from build123d import *

# Parameters (mm, degrees)
SKETCH1_W             = 10
SKETCH1_H             = 10
BOSS_EXTRUDE1_DEPTH   = 2.5
BOSS_EXTRUDE1_2_DEPTH = 2.5
BOSS_EXTRUDE2_DEPTH   = 3
F_2_CLEARANCE_HOLE1_D = 2.9464
FILLET1_R             = 2.5
F_2_CLEARANCE_HOLE2_D = 2.9464
CUT_EXTRUDE1_DEPTH    = 66.097235732
FILLET2_R             = 1
FILLET3_R             = 0.5


with BuildPart() as part:
    # Sketch1 → Boss-Extrude1 (new body)
    with BuildSketch(Plane(origin=(0, 0, 0), x_dir=(1, 0, 0), z_dir=(0, 1, 0))):
        with Locations((-37.51, 0)):
            Rectangle(SKETCH1_W, SKETCH1_H)
    extrude(amount=BOSS_EXTRUDE1_DEPTH)



with BuildPart() as body_2:
    # Sketch1 → Boss-Extrude1 2 (new body)
    with BuildSketch(Plane(origin=(0, 0, 0), x_dir=(1, 0, 0), z_dir=(0, 1, 0))):
        with Locations((37.51, 0)):
            Rectangle(SKETCH1_W, SKETCH1_H)
    extrude(amount=BOSS_EXTRUDE1_2_DEPTH)


with BuildPart() as part_1:
    add(part.part)

    add(body_2.part)  # Boss-Extrude2 merges body 2
    # Sketch2 → Boss-Extrude2 (add)
    with BuildSketch(Plane(origin=(0, 2.5, 0), x_dir=(1, 0, 0), z_dir=(0, 1, 0))):
        with BuildLine():
            Line((-57.51, -5.611149062), (-57.51, 20))
            Line((-57.51, 20), (57.51, 20))
            Line((57.51, 20), (57.51, -5.611149062))
            ThreePointArc((57.51, -5.611149062), (0, -30), (-57.51, -5.611149062))
        make_face()
    extrude(amount=BOSS_EXTRUDE2_DEPTH)

    # #2 Clearance Hole1 (through all)
    with Locations(Plane(origin=(0, 5.5, 0), x_dir=(1, 0, 0), z_dir=(0, 1, 0))):
        with Locations((17.355673654, -24.350342312), (-17.355673654, -24.350342312), (-8, -26), (-52.781944421, 5.448976145), (-45, 0), (45, 0), (52.781944421, 5.448976145), (8, -26)):
            Hole(F_2_CLEARANCE_HOLE1_D / 2)

    # Fillet1
    fillet1_edges = [part_1.edges().sort_by_distance(p)[0] for p in [
        (-57.51, 4, 5.611149062),
        (57.51, 4, 5.611149062),
        (57.51, 4, -20),
        (-57.51, 4, -20),
        (32.51, 1.25, -5),
        (32.51, 1.25, 5),
        (42.51, 1.25, 5),
        (42.51, 1.25, -5),
        (-32.51, 1.25, 5),
        (-42.51, 1.25, 5),
        (-42.51, 1.25, -5),
        (-32.51, 1.25, -5),
    ]]
    fillet(fillet1_edges, radius=FILLET1_R)

    # #2 Clearance Hole2 (through all)
    with Locations(Plane(origin=(0, 5.5, 0), x_dir=(1, 0, 0), z_dir=(0, 1, 0))):
        with Locations((-37.51, 0), (37.51, 0)):
            Hole(F_2_CLEARANCE_HOLE2_D / 2)

    # Sketch7 → Cut-Extrude1 (cut, through all)
    with BuildSketch(Plane(origin=(0, 5.5, 0), x_dir=(1, 0, 0), z_dir=(0, 1, 0))):
        with BuildLine():
            Line((-1, -17.5), (-1, -29.993749756))
            Line((-1, -29.993749756), (0, -30))
            Line((0, -30), (1, -29.993749756))
            Line((1, -29.993749756), (1, -17.5))
            ThreePointArc((1, -17.5), (5.512342988, -17.281974367), (10, -16.762639253))
            Line((10, -16.762639253), (10, -13.727588672))
            ThreePointArc((10, -13.727588672), (5.762621308, -14.249496135), (1.5, -14.489964785))
            Line((1.5, -14.489964785), (0, -15.989964785))
            Line((0, -15.989964785), (-1.5, -14.489964785))
            ThreePointArc((-1.5, -14.489964785), (-5.762621308, -14.249496135), (-10, -13.727588672))
            Line((-10, -13.727588672), (-10, -16.762639253))
            ThreePointArc((-10, -16.762639253), (-5.512342988, -17.281974367), (-1, -17.5))
        make_face()
    extrude(amount=-CUT_EXTRUDE1_DEPTH, mode=Mode.SUBTRACT)


with BuildPart() as cut_extrude1_kept_piece:
    # of the separate pieces the step leaves, the one the design keeps (cut_extrude1_pieces_kept)
    add(part_1.part.solids().sort_by_distance((-57.51, 2.5, 4.590749216))[0])

    # Fillet2
    fillet2_edges = [cut_extrude1_kept_piece.edges().sort_by_distance(p)[0] for p in [
        (10, 4, 13.727588672),
        (10, 4, 16.762639253),
        (1, 4, 29.993749756),
        (-1, 4, 29.993749756),
        (-10, 4, 16.762639253),
        (-1.5, 4, 14.489964785),
        (1.5, 4, 14.489964785),
        (-10, 4, 13.727588672),
    ]]
    fillet(fillet2_edges, radius=FILLET2_R)

    # Fillet3
    fillet3_edges = [cut_extrude1_kept_piece.edges().sort_by_distance(p)[0] for p in [
        (1, 4, 17.5),
        (-1, 4, 17.5),
        (0, 4, 15.989964785),
    ]]
    fillet(fillet3_edges, radius=FILLET3_R)


solid = cut_extrude1_kept_piece.part
Here's how the part is built. I have some questions about the finished solid (model axes, mm). A direction names the side the tool comes from. Coordinates: 2 decimals unless noted, no trailing zeros. Write each loop counter-clockwise with the first axis right and the second up, starting at its lowest first coordinate (ties: lowest second). Pieces come first, ordered by that corner, then holes.
Item 1: On a 3-axis mill with a long thin cutter (end or side, diameter ignored), from which of +Z, -Z, +X, -X, +Y, -Y can I reach the whole of each face in a straight line? I mean faces 5 (the flat face through (37, 1, -5)), 6 (the flat face through (-1, 4, 23)), 7 (the cylindrical face through (-5.374, 4.021, 17.293)), 8 (the cylindrical face through (33.223, 1.268, 4.248)), 9 (the flat face through (37, 1, 5)). Say none if no direction works.
Item 2: I want a section at C-C on z = -12. Write out the boundary of the cut face in (x, y), and give its area (3 significant figures).
Item 3: If we mould it in two halves opening along X, with no side actions, what happens to faces 1 (the cylindrical face through (-33.262, 1.268, -4.287)), 2 (the cylindrical face through (32.081, 3.979, 23.286)), 3 (the flat face through (1, 5.5, -1)), 4 (the flat face through (-42.51, 1, 0))? For each: +X half, -X half, draft (parallel to the pull), parting line (faces both ways), or undercut.
Item 4: If I drill on line 1 (Z direction, x = 8, y = 4.7); line 2 (X direction, y = 4.45, z = -5); line 3 (Y direction, x = -47, z = 8), over which ranges is the centre line in solid material (lowest first)?
Item 5: I want a section at A-A on y = 1.3. Write out the boundary of the cut face in (x, z), and give its area (3 significant figures).
Item 6: Will these pins go through, and if not, where does the flat tip stop? pin 1 (0.5 mm diameter, centred on y = 4.5, z = 15.5, fed in from -X); pin 2 (0.8 mm diameter, centred on x = 37.5, y = 1.5, fed in from -Z); pin 3 (0.9 mm diameter, centred on y = 3.5, z = 24.5, fed in from +X).
Item 7: I want a section at D-D on x = 24. Write out the boundary of the cut face in (y, z).
Item 8: I want a section at B-B on x = -45. Write out the boundary of the cut face in (y, z), and give its area (3 significant figures).
Findings below:
1. face 5: -Z, +X, -X, -Y
1. face 6: +Z, +Y, -Y
1. face 7: +Y, -Y
1. face 8: +Z, -Y
1. face 9: +Z, +X, -X, -Y
2. outline: (-57.51, 2.5) - (57.51, 2.5) - (57.51, 5.5) - (-57.51, 5.5) - close
2. area: 345 mm2
3. face 1: undercut
3. face 2: +X half
3. face 3: draft
3. face 4: -X half
4. line 1: z = -20 to 14.01, 17.03 to 24.53, 27.47 to 29.6
4. line 2: x = -57.51 to -54.19, -51.38 to 51.38, 54.19 to 57.51
4. line 3: y = 2.5 to 5.5
5. outline: (-42.51, -2.5) arc R2.5 ccw to (-40.01, -5) - (-35.01, -5) arc R2.5 ccw to (-32.51, -2.5) - (-32.51, 2.5) arc R2.5 ccw to (-35.01, 5) - (-40.01, 5) arc R2.5 ccw to (-42.51, 2.5) - close; (32.51, -2.5) arc R2.5 ccw to (35.01, -5) - (40.01, -5) arc R2.5 ccw to (42.51, -2.5) - (42.51, 2.5) arc R2.5 ccw to (40.01, 5) - (35.01, 5) arc R2.5 ccw to (32.51, 2.5) - close; hole circle Ø2.95 at (-37.51, 0); hole circle Ø2.95 at (37.51, 0)
5. area: 176 mm2
6. pin 1: stops at x = -46.29
6. pin 2: stops at z = -5
6. pin 3: stops at x = 30.28
7. outline: (2.5, -20) - (5.5, -20) - (5.5, 26.32) - (2.5, 26.32) - close
8. outline: (2.5, -20) - (5.5, -20) - (5.5, -1.47) - (2.5, -1.47) - close; (2.5, 1.47) - (5.5, 1.47) - (5.5, 16.14) - (2.5, 16.14) - close
8. area: 99.6 mm2
